Verification items for this drawing (mm, ordinates from the low corner). Coordinates: 2 decimals unless noted, no trailing zeros. Write each loop counter-clockwise with the first axis right and the second up, starting at its lowest first coordinate (ties: lowest second). Pieces come first, ordered by that corner, then holes. Notation, with made-up numbers: (72, 81) -> (99, 81) arc R34 ccw to (99, 115) -> close; hole circle Ø6 at (-29.75, 81). An arc over 180 degrees is marked (long way). Answer as CSV lines item,"result".
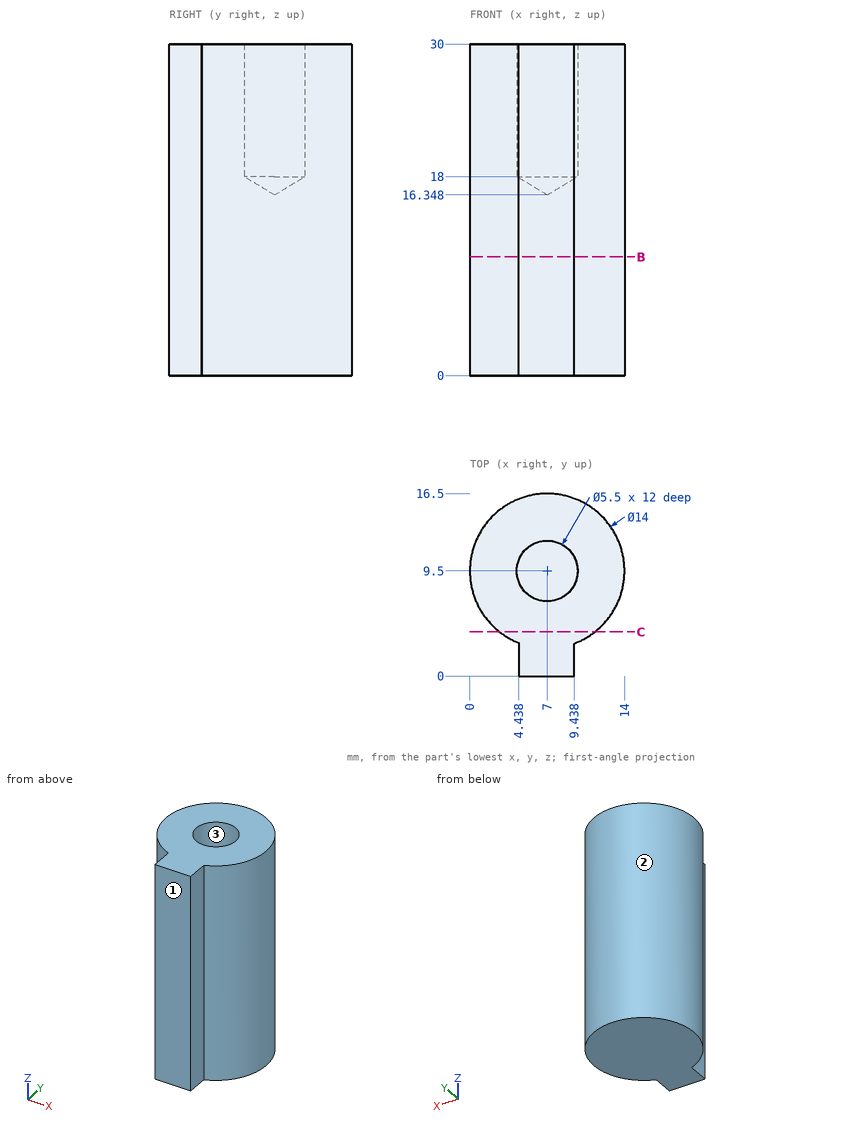
Item 1: Cross-section at C-C, the plane y = 4. Record the cut outline in (x, z), plus the area to 3 significant figures.
Responses:
outline,"(2.67, 0) -> (11.33, 0) -> (11.33, 30) -> (2.67, 30) -> close"
area,"260 mm2"
Item 2: Release check for a two-part mould opening along X. For the marked faces 1, 2 and 3 record: +X half, -X half, draft (parallel to the pull), parting line (faces both ways), or undercut.
Responses:
face 1,"draft"
face 2,"parting line"
face 3,"undercut"
Item 3: Depth check by flat-ended pin: pin 1 Ø2 at (x, y) = (9.5, 9.5) entering from -Z; pin 2 Ø6 at (y, z) = (2, 24) entering from -X; pin 3 Ø2.5 at (y, z) = (1, 19.5) entering from +X; pin 4 Ø0.9 at (y, z) = (1.5, 14.5) entering from -X. Enter the tip coordinate at first touch or a pass-through.
Responses:
pin 1,"stops at z = 0"
pin 2,"stops at x = 1.64"
pin 3,"stops at x = 9.44"
pin 4,"stops at x = 4.44"
Item 4: Thickness scan on probe 1 along Y at (x, z) = (7, 22.75); probe 2 along X at (y, z) = (9.5, 22); probe 3 along Y at (x, z) = (6, 17.75) (1 decimal). Record the ranges inside material, lowest first.
Responses:
probe 1,"y = 0 to 6.75, 12.25 to 16.5"
probe 2,"x = 0 to 4.25, 9.75 to 14"
probe 3,"y = 0 to 7.4, 11.6 to 16.4"
Item 5: Cross-section at B-B, the plane z = 10.75. Record the cut outline in (x, y) (1 decimal), plus the area to 3 significant figures.
Responses:
outline,"(4.4, 0) -> (9.4, 0) -> (9.4, 2.9) arc R7 ccw (long way) to (4.4, 3) -> close"
area,"167 mm2"
